Part model, mm, in its own coordinate system. A direction names the side the tool comes from. Give positions to 0.01 mm unless a question says otherwise; leave off trailing zeros. Write each loop counter-clockwise with the first axis right and the second up, starting at its lowest first coordinate (ties: lowest second). Pieces come first, ordered by that corner, then holes. Notation, with made-up numbers: M -22,-35.75 L 7,-35.75 A34 ccw 7,-1.75 Z; hole C 16.25,-6 d10. An arc over 180 degrees is marked long. Use CSV: the item, a comma, the result in double quotes. Start each with the question number.
1. Band-saw the part on D-D, the plane z = 13.7. List the corners of the cut face in (x, y), then the cut area to 3 significant figures.
2. Drop a flat-ended pin along its axis: pin 1 Ø4.5 at (x, y) = (-15, 0) entering from +Z. Give the stop position or say it passes through.
3. Mould opens along Y. For faces 3 (the face through (0, 5.5, 15)), 4 (the face through (3.5, -2.5, 14.8)), 5 (the face through (0, 3, 13)) say: pulls with the +Y half, pulls with the -Y half, needs draft (parallel to the pull), parting line crosses it, or undercut.
4. 3-axis set-ups, long thin cutter, end or side, ignore diameter. For faces 1 (the face through (-20, 0, 15)), 2 (the face through (-4.5, 0, 15)): which of +Z, -Z, +X, -X, +Y, -Y reach the whole face in a straight line?
5. Band-saw the part on A-A, the plane y = 0. List the corners of the cut face in (x, z), then the cut area to 3 significant figures.
6. Band-saw the part on B-B, the plane z = 16.05. List the corners of the cut face in (x, y), then the cut area to 3 significant figures.
7. Band-saw the part on C-C, the plane x = 3.5. List the corners of the cut face in (y, z).
8. Drill centre lines: line 1 along Y through (x, z) = (15, 14.25); line 2 along X through (y, z) = (-1, 16.25); line 3 along X through (y, z) = (0.75, 13.35). Where is each one in solid material? Low to high. Write a range as from..to.
from build123d import *

# Parameters (mm, degrees)
ESQUISSE1_W                                        = 40
ESQUISSE1_H                                        = 11
ESQUISSE1_R                                        = 4
BOSS_EXTRU_1_DEPTH                                 = 9.51
ESQUISSE16_W                                       = 40
ESQUISSE16_H                                       = 11
BOSS_EXTRU_2_DEPTH                                 = 7
D_GAGEMENT_M32_D                                   = 2.5
ENL_V_MAT_EXTRU_1_DEPTH                            = 7
CHAMBRAGE_POUR_VIS_T_TE_RONDE_BOMB_E_M_D           = 3.4
CHAMBRAGE_POUR_VIS_T_TE_RONDE_BOMB_E_M_CBORE_D     = 6
CHAMBRAGE_POUR_VIS_T_TE_RONDE_BOMB_E_M_CBORE_DEPTH = 2.4
FRAISAGE_POUR_VIS_T_TE_FRAIS_E_M31_D               = 3.4
FRAISAGE_POUR_VIS_T_TE_FRAIS_E_M31_DEPTH           = 6
FRAISAGE_POUR_VIS_T_TE_FRAIS_E_M31_CSINK_D         = 6.3
FRAISAGE_POUR_VIS_T_TE_FRAIS_E_M31_CSINK_ANGLE     = 90
FRAISAGE_POUR_VIS_T_TE_FRAIS_E_M31_TIP             = 1.021463052
ESQUISSE33_W                                       = 53.617438424
ESQUISSE33_H                                       = 31.43157248
ENL_V_MAT_EXTRU_4_DEPTH                            = 13


with BuildPart() as part:
    # Esquisse1 → Boss.-Extru.1 (new body)
    with BuildSketch(Plane.XY):
        Rectangle(ESQUISSE1_W, ESQUISSE1_H)
        Circle(ESQUISSE1_R, mode=Mode.SUBTRACT)
    extrude(amount=BOSS_EXTRU_1_DEPTH)

    # Esquisse16 → Boss.-Extru.2 (add)
    with BuildSketch(Plane.XY.offset(9.51)):
        Rectangle(ESQUISSE16_W, ESQUISSE16_H)
    extrude(amount=BOSS_EXTRU_2_DEPTH)

    # Dégagement M32 (through all)
    with Locations(Plane.XY.offset(16.51)):
        with Locations((0, 0)):
            Hole(D_GAGEMENT_M32_D / 2)

    # Esquisse19 → Enlèv. mat.-Extru.1 (cut)
    with BuildSketch(Plane.XY.offset(16.51)):
        with BuildLine():
            Line((-2.5, 1.5), (-2.5, -1.5))
            ThreePointArc((-2.5, -1.5), (-3.5, -2.5), (-4.5, -1.5))
            Line((-4.5, -1.5), (-4.5, 1.5))
            ThreePointArc((-4.5, 1.5), (-3.5, 2.5), (-2.5, 1.5))
        make_face()
        with BuildLine():
            Line((4.5, 1.5), (4.5, -1.5))
            ThreePointArc((4.5, -1.5), (3.5, -2.5), (2.5, -1.5))
            Line((2.5, -1.5), (2.5, 1.5))
            ThreePointArc((2.5, 1.5), (3.5, 2.5), (4.5, 1.5))
        make_face()
    extrude(amount=-ENL_V_MAT_EXTRU_1_DEPTH, mode=Mode.SUBTRACT)

    # Chambrage pour vis _ t_te ronde bomb_e M (through all)
    with Locations(Plane(origin=(0, 5.5, 0), x_dir=(1, 0, 0), z_dir=(0, 1, 0))):
        with Locations((14, -6.51), (-14, -6.51)):
            CounterBoreHole(CHAMBRAGE_POUR_VIS_T_TE_RONDE_BOMB_E_M_D / 2, CHAMBRAGE_POUR_VIS_T_TE_RONDE_BOMB_E_M_CBORE_D / 2, CHAMBRAGE_POUR_VIS_T_TE_RONDE_BOMB_E_M_CBORE_DEPTH)

    # Fraisage pour vis à tête fraisée M31
    with Locations(Plane.XY.offset(16.51)):
        with Locations((-15, 0), (15, 0)):
            CounterSinkHole(FRAISAGE_POUR_VIS_T_TE_FRAIS_E_M31_D / 2, FRAISAGE_POUR_VIS_T_TE_FRAIS_E_M31_CSINK_D / 2, depth=FRAISAGE_POUR_VIS_T_TE_FRAIS_E_M31_DEPTH, counter_sink_angle=FRAISAGE_POUR_VIS_T_TE_FRAIS_E_M31_CSINK_ANGLE)
            with Locations((0, 0, -(FRAISAGE_POUR_VIS_T_TE_FRAIS_E_M31_DEPTH + FRAISAGE_POUR_VIS_T_TE_FRAIS_E_M31_TIP / 2))):  # 118° drill point
                Cone(0, FRAISAGE_POUR_VIS_T_TE_FRAIS_E_M31_D / 2, FRAISAGE_POUR_VIS_T_TE_FRAIS_E_M31_TIP, mode=Mode.SUBTRACT)

    # Esquisse33 → Enlèv. mat.-Extru.4 (cut)
    with BuildSketch(Plane(origin=(0, 0, 0), x_dir=(-1, 0, 0), z_dir=(0, 0, -1))):
        Rectangle(ESQUISSE33_W, ESQUISSE33_H)
    extrude(amount=-ENL_V_MAT_EXTRU_4_DEPTH, mode=Mode.SUBTRACT)


solid = part.part
Output:
1,outline,"M -20,-5.5 L 20,-5.5 L 20,5.5 L -20,5.5 Z; hole C -15,0 d3.4; hole M -4.5,-1.5 A1 ccw -2.5,-1.5 L -2.5,1.5 A1 ccw -4.5,1.5 Z; hole C 0,0 d2.5; hole M 2.5,-1.5 A1 ccw 4.5,-1.5 L 4.5,1.5 A1 ccw 2.5,1.5 Z; hole C 15,0 d3.4"
1,area,"399 mm²"
2,pin 1,"stops at z = 15.61"
3,face 3,"pulls with the +Y half"
3,face 4,"undercut"
3,face 5,"needs draft"
4,face 1,"+Z, -Z, -X, +Y, -Y"
4,face 2,"+Z, -Z"
5,outline,"M -20,13 L -16.7,13 L -16.7,15.06 L -18.15,16.51 L -20,16.51 Z; M -13.3,13 L -4.5,13 L -4.5,16.51 L -11.85,16.51 L -13.3,15.06 Z; M -2.5,13 L -1.25,13 L -1.25,16.51 L -2.5,16.51 Z; M 1.25,13 L 2.5,13 L 2.5,16.51 L 1.25,16.51 Z; M 4.5,13 L 13.3,13 L 13.3,15.06 L 11.85,16.51 L 4.5,16.51 Z; M 16.7,13 L 20,13 L 20,16.51 L 18.15,16.51 L 16.7,15.06 Z"
5,area,"89.5 mm²"
6,outline,"M -20,-5.5 L 20,-5.5 L 20,5.5 L -20,5.5 Z; hole C -15,0 d5.38; hole M -4.5,-1.5 A1 ccw -2.5,-1.5 L -2.5,1.5 A1 ccw -4.5,1.5 Z; hole C 0,0 d2.5; hole M 2.5,-1.5 A1 ccw 4.5,-1.5 L 4.5,1.5 A1 ccw 2.5,1.5 Z; hole C 15,0 d5.38"
6,area,"371 mm²"
7,outline,"M -5.5,13 L -2.5,13 L -2.5,16.51 L -5.5,16.51 Z; M 2.5,13 L 5.5,13 L 5.5,16.51 L 2.5,16.51 Z"
8,line 1,"y = -5.5..-1.7, 1.7..5.5"
8,line 2,"x = -20..-17.71, -12.29..-4.5, -2.5..-0.75, 0.75..2.5, 4.5..12.29, 17.71..20"
8,line 3,"x = -20..-16.53, -13.47..-4.5, -2.5..-1, 1..2.5, 4.5..13.47, 16.53..20"
